Work out the finished part from the listing and answer in its coordinate system (mm). A direction names the side the tool comes from. Give positions to 0.01 mm unless a question says otherwise; leave off trailing zeros. Loops run counter-clockwise (first coordinate to the right, second up) from the corner with the lowest first, then second, coordinate; pieces in that order, holes last. Notation, with made-up numbers: M 51,64.25 L 59,64.25 A24 ccw 59,85.25 Z; hole C 86,1 d1. An arc over 180 degrees is marked long. Write item = value, one per line. Start each with the question number.
1. For faces 1 (the face through (72.205, 49.226, 35.496)), 2 (the face through (-10.13, 1.38, 60.12)), 3 (the face through (-27, 9, 21.633)), 4 (the face through (-58.134, 9.484, 16.242)), 5 (the face through (6.912, 9.292, 35.558)), determine the directions among +Z, -Z, +X, -X, +Y, -Y from which every point of the face is accessible in a straight line to the end or side of a thin tool.
2. Flat-ended cylindrical pins translate along their axes: pin 1 Ø2 at (y, z) = (115, 13.5) entering from -X; pin 2 Ø1.5 at (y, z) = (33.5, 59) entering from +X; pin 3 Ø0.6 at (y, z) = (15.5, 50.5) entering from +X; pin 4 Ø10 at (x, y) = (49.5, 78.5) entering from +Z. Find the tip coordinate at first contact, or state that the pin passes through.
3. Section C-C on z = 26.5 is taken. Determine the outline of the cut face in (x, y).
4. Section A-A on x = -48 is taken. Determine the outline of the cut face in (y, z), plus the area to 3 significant figures.
5. The mould has two halves that part along Z. Classify faces 6 (the face through (24.59, -7.86, 5.48)), 7 (the face through (71.822, 143.543, 15.522)), 8 (the face through (-37, 4, 11)): released by +Z, released by -Z, zero draft, split by the parting line, or undercut.
6. Section B-B on z = 14.5 is taken. Determine the outline of the cut face in (x, y).
7. Section D-D on x = 15.5 is taken. Give the number of separate pieces and of enclosed holes in the cut face, plus the area to 3 significant figures.
8. Consider L1, parallel to Z at x = -8, y = 8.5; L2, parallel to Z at x = 50.5, y = 92.5; L3, parallel to Z at x = 43.5, y = 51.5. Determine where each line is inside the solid, lowest interval first. Write a range as [from, to].
```python
from build123d import *

# Parameters (mm, degrees)
BOSS_EXTRUDE1_DEPTH = 72
CUT_EXTRUDE1_DEPTH  = 72
SKETCH4_W           = 26
SKETCH4_H           = 28.511973983
SKETCH4_W_2         = 24
CUT_EXTRUDE2_DEPTH  = 72
CUT_EXTRUDE3_DEPTH  = 72
CUT_EXTRUDE4_DEPTH  = 72
SKETCH10_R          = 4
CUT_EXTRUDE5_DEPTH  = 72
SKETCH9_R           = 4
CUT_EXTRUDE6_DEPTH  = 72
SKETCH11_R          = 2.5
CUT_EXTRUDE7_DEPTH  = 100
SKETCH15_R          = 5
CUT_EXTRUDE9_DEPTH  = 20


# Read off the part's stored shape, not the designer's step: Boss-Extrude1
with BuildPart() as part:
    # Boss-Extrude1 outline → Boss-Extrude1 (new body)
    with BuildSketch(Plane.XY):
        with BuildLine():
            Line((62.494511824, 50.937989443), (82.190666884, 47.46502589))
            Line((82.190666884, 47.46502589), (93.534081641, 111.796727777))
            ThreePointArc((93.534081641, 111.796727777), (71.22719332, 143.654265871), (39.369655226, 121.347377549))
            Line((39.369655226, 121.347377549), (23.783847578, 32.955869992))
            Line((23.783847578, 32.955869992), (-34.13991608, 32.955869992))
            ThreePointArc((-34.13991608, 32.955869992), (-58.13991608, 8.955869992), (-34.13991608, -15.044130008))
            Line((-34.13991608, -15.044130008), (50.86008392, -15.044130008))
            Line((50.86008392, -15.044130008), (62.494511824, 50.937989443))
        make_face()
    extrude(amount=BOSS_EXTRUDE1_DEPTH)

    # Sketch3 → Cut-Extrude1 (cut)
    with BuildSketch(Plane(origin=(0, 32.955869992, 0), x_dir=(1, 0, 0), z_dir=(0, 1, 0))):
        Polygon((-9.823766264, 0), (-16.174619225, -11), (-58.13991608, -11), (-58.13991608, 0), align=None)
        Polygon((-9.54918364, -72), (-15.900036601, -61), (-58.13991608, -61), (-58.13991608, -72), align=None)
    extrude(amount=-CUT_EXTRUDE1_DEPTH, mode=Mode.SUBTRACT)

    # Sketch4 → Cut-Extrude2 (cut)
    with BuildSketch(Plane(origin=(0, 32.955869992, 0), x_dir=(1, 0, 0), z_dir=(0, 1, 0))):
        with Locations((-21.13991608, -35.889301659)):
            Rectangle(SKETCH4_W, SKETCH4_H)
        with Locations((-46.13991608, -35.889301659)):
            Rectangle(SKETCH4_W_2, SKETCH4_H)
        with BuildLine():
            ThreePointArc((-8.13991608, -20.833314667), (6.916070911, -35.889301658), (-8.13991608, -50.94528865))
            Line((-8.13991608, -50.94528865), (-8.13991608, -20.833314667))
        make_face()
    extrude(amount=-CUT_EXTRUDE2_DEPTH, mode=Mode.SUBTRACT)

    # Sketch5 → Cut-Extrude3 (cut)
    with BuildSketch(Plane(origin=(71.595317547, -12.624186176, 0), x_dir=(0, 0, -1), z_dir=(0.9848077530122087, -0.173648177666927, 0))):
        Polygon((-72, 82.273588595), (-61.318633323, 88.440478521), (-61.318633323, 153.840307103), (-72, 153.840307103), align=None)
        Polygon((0, 82.273588595), (-10.681366677, 88.440478521), (-10.681366677, 153.840307103), (0, 153.840307103), align=None)
    extrude(amount=-CUT_EXTRUDE3_DEPTH, mode=Mode.SUBTRACT)

    # Sketch7 → Cut-Extrude4 (cut)
    with BuildSketch(Plane(origin=(71.595317547, -12.624186176, 0), x_dir=(0, 0, -1), z_dir=(0.9848077530122087, -0.173648177666927, 0))):
        with BuildLine():
            Line((-51.5, 97.883463974), (-51.5, 153.840307103))
            Line((-51.5, 153.840307103), (-20.5, 153.840307103))
            Line((-20.5, 153.840307103), (-20.5, 97.883463974))
            ThreePointArc((-20.5, 97.883463974), (-36, 77.914837007), (-51.5, 97.883463974))
        make_face()
    extrude(amount=-CUT_EXTRUDE4_DEPTH, mode=Mode.SUBTRACT)

    # Sketch10 → Cut-Extrude5 (cut)
    with BuildSketch(Plane(origin=(0, 0, 10.681366677), x_dir=(-1, 0, 0), z_dir=(0, 0, -1))):
        with Locations((-66.451868434, 116.572052663)):
            Circle(SKETCH10_R)
    extrude(amount=-CUT_EXTRUDE5_DEPTH, mode=Mode.SUBTRACT)

    # Sketch9 → Cut-Extrude6 (cut)
    with BuildSketch(Plane(origin=(0, 0, 11), x_dir=(-1, 0, 0), z_dir=(0, 0, -1))):
        with Locations((34.13991608, 8.955869992)):
            Circle(SKETCH9_R)
    extrude(amount=-CUT_EXTRUDE6_DEPTH, mode=Mode.SUBTRACT)

    # Sketch11 → Cut-Extrude7 (cut)
    with BuildSketch(Plane(origin=(51.899162487, -9.151222623, 0), x_dir=(0, 0, -1), z_dir=(0.9848077530122088, -0.17364817766692606, 0))):
        with Locations(Location((-7, -1.483814981, 0), (0, 0, 90))):
            Circle(SKETCH11_R)
        with Locations(Location((-65, -1.483814981, 0), (0, 0, 90))):
            Circle(SKETCH11_R)
        with Locations(Location((-7, 56.516185019, 0), (0, 0, 90))):
            Circle(SKETCH11_R)
        with Locations(Location((-65, 56.516185019, 0), (0, 0, 90))):
            Circle(SKETCH11_R)
    extrude(amount=-CUT_EXTRUDE7_DEPTH, mode=Mode.SUBTRACT)

    # Sketch15 → Cut-Extrude9 (cut)
    with BuildSketch(Plane(origin=(-21.961418989, 3.872390702, 0), x_dir=(0, 0, 1), z_dir=(-0.9848077530122088, 0.17364817766692614, 0))):
        with Locations(Location((7, -1.483814981, 0), (0, 0, 270))):
            Circle(SKETCH15_R)
        with Locations(Location((65, -1.483814981, 0), (0, 0, 270))):
            Circle(SKETCH15_R)
    extrude(amount=-CUT_EXTRUDE9_DEPTH, mode=Mode.SUBTRACT)


solid = part.part
```
Verdict:
q1.face_1 = +Z, -Z, -Y
q1.face_2 = none
q1.face_3 = -X, +Y, -Y
q1.face_4 = +Z, -Z, -X
q1.face_5 = +Y, -Y
q2.pin_1 = 38.07
q2.pin_2 = 59.55
q2.pin_3 = 56.3
q2.pin_4 = 72
q3.outline = M 3.63,-15.04 L 50.86,-15.04 L 62.49,50.94 L 82.19,47.47 L 85.67,67.19 L 31.5,76.74 L 23.78,32.96 L 3.63,32.96 Z
q4.outline = M -10.64,11 L 28.55,11 L 28.55,21.63 L -10.64,21.63 Z; M -10.64,50.15 L 28.55,50.15 L 28.55,61 L -10.64,61 Z
q4.area = 842 mm2
q5.face_6 = undercut
q5.face_7 = zero draft
q5.face_8 = released by -Z
q6.outline = M -34.14,-15.04 L 50.86,-15.04 L 62.49,50.94 L 82.19,47.47 L 93.53,111.8 A27.5 ccw 39.37,121.35 L 23.78,32.96 L -34.14,32.96 A24 ccw Z; hole C -34.14,8.96 d8; hole C 66.45,116.57 d8
q7.separate_pieces = 1
q7.enclosed_holes = 2
q7.area = 3,420 mm2
q8.L1 = [0, 20.83], [50.94, 72]
q8.L2 = [10.68, 20.5], [51.5, 61.32]
q8.L3 = [0, 5.22], [8.78, 63.22], [66.78, 72]
